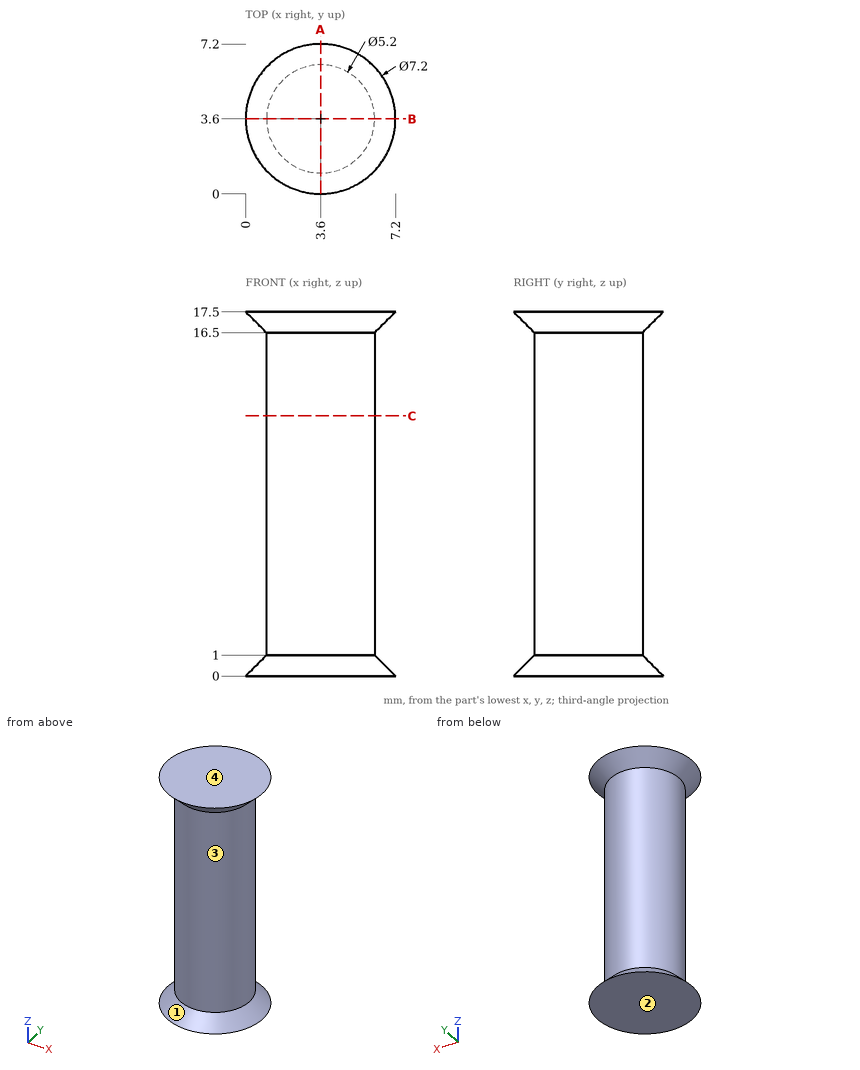
Here's the drawing with two shaded views (mm, measured from the low corner). I have some questions. Round coordinates to 2 decimals unless told otherwise and drop trailing zeros. Order: outer loops, then holes, each group sorted by start corner. A loop starts at its lowest first (then second) coordinate and runs counter-clockwise, first axis right, second up. Notation, with made-up numbers: (-27, 34.25) -> (-1, 34.25) arc R29 ccw to (-1, 71.25) -> close; hole circle Ø1 at (-4.5, 3.5). An arc over 180 degrees is marked (long way). Use a Markdown table: item, result. Add a question column.
(1) I need wall thicknesses on line 1 along Z through (x, y) = (6.75, 3.5); line 2 along Z through (x, y) = (5.25, 0.75); line 3 along Y through (x, z) = (5.5, 9.5). Which ranges of each line are inside material? Lowest first, please.
(2) For pin 1 Ø1 at (y, z) = (5, 13.5) entering from -X; pin 2 Ø3 at (x, z) = (3.5, 3) entering from +Y; pin 3 Ø2 at (y, z) = (2.5, 14.5) entering from -X, each with a flat end and sliding along its axis, tell me the tip position at first contact or that it passes through.
(3) Suppose I cut it at A-A, the plane x = 3.6. Please give me the cut outline in (y, z).
(4) If we mould it in two halves opening along Z, with no side actions, what happens to the marked faces 1, 2, 3 and 4? For each: released by +Z, released by -Z, zero draft, split by the parting line, or undercut.
(5) Suppose I cut it at C-C, the plane z = 12.5. Please give me the cut outline in (x, y).
Verdict:
| question | item | result |
|---|---|---|
| 1 | line 1 | 0 to 0.45, 17.05 to 17.5 |
| 1 | line 2 | 0 to 0.31, 17.19 to 17.5 |
| 1 | line 3 | 1.83 to 5.37 |
| 2 | pin 1 | x = 1.16 |
| 2 | pin 2 | y = 6.2 |
| 2 | pin 3 | x = 1 |
| 3 | outline | (0, 0) -> (7.2, 0) -> (6.2, 1) -> (6.2, 16.5) -> (7.2, 17.5) -> (0, 17.5) -> (1, 16.5) -> (1, 1) -> close |
| 4 | face 1 | undercut |
| 4 | face 2 | released by -Z |
| 4 | face 3 | undercut |
| 4 | face 4 | released by +Z |
| 5 | outline | circle Ø5.2 at (3.6, 3.6) |
